Work out the finished part from the listing and answer in its coordinate system (mm). A direction names the side the tool comes from. Give positions to 0.01 mm unless a question says otherwise; leave off trailing zeros. Order: outer loops, then holes, each group sorted by start corner. A loop starts at its lowest first (then second) coordinate and runs counter-clockwise, first axis right, second up. Notation, with made-up numbers: (22, 6.25) - (56, 6.25) arc R15 ccw to (56, 31.25) - close; hole circle Ø1 at (42, -28.75). An arc over 180 degrees is marked (long way). Put each result on its own line as item: value.
Autodesk Inventor part; units mm, degrees
ref_plane "YZ Plane" through (0, 0, 0) normal (1, 0, 0) x (0, 1, 0)
ref_plane "XZ Plane" through (0, 0, 0) normal (0, 1, 0) x (-1, 0, 0)
ref_plane "XY Plane" through (0, 0, 0) normal (0, 0, 1) x (1, 0, 0)
sketch "Эскиз1" plane through (0, 0, 0) normal (0, 0, 1) x (1, 0, 0)
  line L0 (-75.6484, -106.9824) -> (60.0028, -106.9824)
  line L1 (60.0028, 113.8664) -> (-75.6484, 113.8664)
  line L2 (-75.6484, -71.558) -> (-75.6484, 58.442)
  line L3 (60.0028, -71.558) -> (60.0028, 78.442)
  line L4 (63.0028, -109.9824) -> (-78.6484, -109.9824)
  line L5 (-78.6484, -109.9824) -> (-78.6484, 116.8664)
  line L6 (-78.6484, 116.8664) -> (63.0028, 116.8664)
  line L7 (63.0028, 116.8664) -> (63.0028, -109.9824)
  line L8 (60.0028, -106.9824) -> (-75.6484, -106.9824)
  line L9 (-75.6484, -106.9824) -> (-75.6484, 113.8664)
  line L10 (-75.6484, 113.8664) -> (60.0028, 113.8664)
  line L11 (60.0028, 113.8664) -> (60.0028, -106.9824)
  point P0 (0, 0)
  dimension "d0" = 3
  dimension "d1" = 3
  dimension "d2" = 3
  dimension "d3" = 3
extrude "Выдавливание1" add sketch "Эскиз1" along normal blind 60
sketch "Эскиз2" plane through (63.0028, -109.9824, 0) normal (1, 0, 0) x (0, 0, -1)
  point P0 (0, 109.9824)
sketch "Эскиз3" plane through (0, 0, 0) normal (0, 0, -1) x (-1, 0, 0)
  point P0 (0, 0)
sketch "Эскиз4" plane through (63.0028, -109.9824, 0) normal (1, 0, 0) x (0, 0, -1)
  line L0 (-8, 38.4244) -> (-8, 3)
  line L1 (-8, 3) -> (-8, 38.4244)
  line L2 (0.0001, 223.8488) -> (0, 188.4244)
  line L3 (-8, 188.4244) -> (-7.9999, 223.8488)
  line L4 (0, 223.8488) -> (0, 3)
  line L5 (-8, 38.4244) -> (0, 38.4244)
  line L6 (0, 38.4244) -> (0, 3)
  line L7 (0, 3) -> (-8, 3)
  line L8 (-8, 3) -> (-8, 38.4244)
  line L9 (-7.9999, 223.8488) -> (0, 223.8488)
  line L10 (0, 223.8488) -> (0, 188.4244)
  line L11 (0, 188.4244) -> (-7.9999, 188.4244)
  line L12 (-7.9999, 188.4244) -> (-7.9999, 223.8488)
  point P0 (0, 109.9824)
extrude "Выдавливание2" cut sketch "Эскиз4" against normal blind 239.25
sketch "Эскиз5" plane through (0, 0, 60) normal (0, 0, 1) x (1, 0, 0)
  line L0 (73.8028, -108.2777) -> (32.8028, -108.2777)
  line L1 (63.0028, 116.8664) -> (-78.6484, 116.8664)
  line L2 (-78.6484, 116.8664) -> (-78.6484, -109.9824)
  line L3 (-78.6484, -109.9824) -> (63.0028, -109.9824)
  line L4 (63.0028, -109.9824) -> (63.0028, 116.8664)
  line L5 (60.0028, 113.8664) -> (60.0028, -106.9824)
  line L6 (60.0028, -106.9824) -> (-75.6484, -106.9824)
  line L7 (-75.6484, -106.9824) -> (-75.6484, 113.8664)
  line L8 (-75.6484, 113.8664) -> (60.0028, 113.8664)
  line L9 (60.0028, -106.9824) -> (-75.6484, -106.9824)
  line L10 (-75.6484, 113.8664) -> (60.0028, 113.8664)
  line L11 (56.3016, -106.9824) -> (26.1407, -106.9824)
  line L12 (26.1407, -106.9824) -> (26.1407, 113.8664)
  line L13 (26.1407, 113.8664) -> (56.3016, 113.8664)
  line L14 (56.3016, 113.8664) -> (56.3016, -106.9824)
  line L15 (5.2877, -106.9824) -> (-25.8022, -106.9824)
  line L16 (-25.8022, -106.9824) -> (-25.8022, 113.8664)
  line L17 (-25.8022, 113.8664) -> (5.2877, 113.8664)
  line L18 (5.2877, 113.8664) -> (5.2877, -106.9824)
  line L19 (-48.9301, -106.9824) -> (-75.6484, -106.9824)
  line L20 (-75.6484, -106.9824) -> (-75.6484, 111.5008)
  line L21 (-75.6484, 111.5008) -> (-48.9301, 111.5008)
  line L22 (-48.9301, 111.5008) -> (-48.9301, -106.9824)
  line L23 (-75.6484, -106.9824) -> (-75.6484, 113.8664)
  line L24 (-75.6484, -32.9455) -> (-73.4662, -32.9455)
  line L25 (-73.4662, -32.9455) -> (-73.4662, -24.8216)
  line L26 (-73.4662, -24.8216) -> (-75.6484, -24.8216)
  line L27 (-75.6484, -24.8216) -> (-75.6484, -32.9455)
  line L28 (-75.6484, 29.4025) -> (-73.4662, 29.4025)
  line L29 (-73.4662, 29.4025) -> (-73.4662, 36.4767)
  line L30 (-73.4662, 36.4767) -> (-75.6484, 36.4767)
  line L31 (-75.6484, 36.4767) -> (-75.6484, 29.4025)
  point P0 (0, 0)
extrude "Выдавливание3" add sketch "Эскиз5" along normal blind 5 contours L4 L3 L2 L1 | L14 L6 L12 L8 | L18 L6 L16 L8 | L6 L7 L24 L25 L26 L28 L29 L30 L21 L22
sketch "Эскиз6" plane through (0, 0, 65) normal (0, 0, 1) x (1, 0, 0)
  line L0 (-48.9301, 111.5008) -> (-75.6484, 111.5008)
  line L1 (-75.6484, 111.5008) -> (-75.6484, 113.8664)
  line L2 (-48.9301, 111.5008) -> (-75.6484, 111.5008)
  line L3 (-75.6484, 111.5008) -> (-75.6484, 113.8664)
  line L4 (-75.6484, 113.8664) -> (-48.9301, 113.8664)
  line L5 (-48.9301, 113.8664) -> (-48.9301, 111.5008)
  point P0 (0, 0)
extrude "Выдавливание4" add sketch "Эскиз6" against normal blind 5
sketch "Эскиз7" plane through (-78.6484, -71.558, 0) normal (-1, 0, 0) x (0, 0, 1)
  point P0 (0, 71.558)
sketch "Эскиз8" plane through (-78.6484, 116.8664, 0) normal (0, 1, 0) x (1, 0, 0)
  line L0 (85.4799, -9.5) -> (62.4799, -9.5)
  line L1 (74.1362, -4.2225) -> (79.8964, -4.2225)
  line L2 (141.6512, 0) -> (0, 0)
  line L3 (85.4799, -9.5) -> (64.1362, -9.5)
  line L4 (64.1362, -9.5) -> (64.1362, 0)
  line L5 (64.1362, 0) -> (85.4799, 0)
  line L6 (85.4799, 0) -> (85.4799, -9.5)
  line L7 (64.1362, -9.5) -> (89.8964, -9.5)
  line L8 (89.8964, -9.5) -> (89.8964, 0)
  line L9 (89.8964, 0) -> (64.1362, 0)
  line L10 (64.1362, 0) -> (64.1362, -9.5)
  point P0 (78.6484, 0)
  dimension "d12" = 10
  dimension "d13" = 5.584
  dimension "d14" = 10
extrude "Выдавливание5" cut sketch "Эскиз8" against normal blind 5
sketch "Эскиз9" plane through (63.0028, -71.558, 0) normal (1, 0, 0) x (0, 0, -1)
  line L0 (-65, -38.4244) -> (-65, 188.4244)
  arc A0 (-65, 188.4244) -> (-65, -38.4244) centre (307.5062, 75) ccw
  line L1 (0, -38.4244) -> (-65, -38.4244)
  line L2 (-65, -38.4244) -> (-65, -28.4244)
  line L3 (-65, -28.4244) -> (-65, 178.4244)
  arc A1 (-65, 178.4244) -> (-65, -28.4244) centre (307.5062, 75) ccw
  point P0 (0, 71.558)
  dimension "d17" = 10
  dimension "d18" = 10
extrude "Выдавливание6" add sketch "Эскиз9" against normal blind 141.651 contours A0 L0 A1
sketch "Эскиз10" plane through (63.0028, -71.558, 0) normal (1, 0, 0) x (0, 0, -1)
  arc A0 (-65, 178.4244) -> (-65, -28.4244) centre (307.5062, 75) ccw
  line L0 (-65, -28.4244) -> (-65, 178.4244)
  point P0 (0, 71.558)
extrude "Выдавливание7" add sketch "Эскиз10" against normal blind 3
sketch "Эскиз11" plane through (-78.6484, -71.558, 0) normal (-1, 0, 0) x (0, 0, 1)
  arc A0 (65, -28.4244) -> (65, 178.4244) centre (-307.5062, 75) ccw
  line L0 (65, 188.4244) -> (65, -38.4244)
  point P0 (0, 71.558)
extrude "Выдавливание8" add sketch "Эскиз11" against normal blind 3
sketch "Эскиз12" plane through (-78.6484, -109.9824, 0) normal (0, -1, 0) x (1, 0, 0)
  spline S0 degree 3 poles (75.9334, 40.3738) (75.8831, 40.8501) (75.7622, 41.3112) (75.3324, 42.3118) (75.0359, 42.7084) (74.4654, 43.3771) (73.9913, 43.782) (72.8589, 44.371) (72.2642, 44.5465) (71.3446, 44.633) (71.0335, 44.6318) (70.0476, 44.5299) (69.4546, 44.3267) (68.4476, 43.7801) (67.9673, 43.407) (67.0987, 42.3576) (66.8298, 41.785) (66.5793, 40.9818) (66.515, 40.667) (66.4421, 39.9332) (66.4622, 39.6005) (66.486, 39.3756) knots -0.649055 -0.649055 -0.649055 -0.649055 -0.611574 -0.611574 -0.563504 -0.563504 -0.482019 -0.482019 -0.407033 -0.407033 -0.368981 -0.368981 -0.286973 -0.286973 -0.207347 -0.207347 -0.121004 -0.121004 -0.067856 -0.067856 0 0 0 0
  spline S1 degree 3 poles (66.486, 39.3756) (66.5097, 39.1507) (66.5596, 38.8211) (66.7843, 38.1188) (66.913, 37.8244) (67.3257, 37.0912) (67.7084, 36.5875) (68.7772, 35.7428) (69.3247, 35.4783) (70.4238, 35.1543) (71.0461, 35.0795) (72.0316, 35.1858) (72.3361, 35.2497) (73.2173, 35.5265) (73.7622, 35.8224) (74.7465, 36.635) (75.1255, 37.13) (75.5436, 37.9033) (75.7507, 38.353) (75.9619, 39.4214) (75.9837, 39.8976) (75.9334, 40.3738) knots -2.488 -2.488 -2.488 -2.488 -2.22789 -2.22789 -2.024159 -2.024159 -1.693184 -1.693184 -1.387958 -1.387958 -1.073596 -1.073596 -0.927734 -0.927734 -0.640291 -0.640291 -0.327938 -0.327938 -0.143673 -0.143673 0 0 0 0
  point P0 (78.6484, 0)
extrude "Выдавливание9" cut sketch "Эскиз12" against normal blind 3
sketch "Эскиз13" plane through (-78.6484, 116.8664, 65) normal (0, 1, 0) x (1, 0, 0)
  line L0 (49.8619, 5.8292) -> (89.8619, 5.8292)
  line L1 (89.8619, 37.7292) -> (49.8619, 37.7292)
  line L2 (101.9119, 18.2982) -> (101.9119, 14.2982)
  line L3 (101.9119, 29.2602) -> (101.9119, 25.2602)
  line L4 (77.7841, 5.8292) -> (67.7841, 5.8292)
  line L5 (67.7841, 5.8292) -> (67.7841, 2.8292)
  line L6 (67.7841, 2.8292) -> (77.7841, 2.8292)
  line L7 (77.7841, 2.8292) -> (77.7841, 5.8292)
  line L8 (77.7841, 37.7292) -> (67.7841, 37.7292)
  line L9 (67.7841, 37.7292) -> (67.7841, 40.7292)
  line L10 (67.7841, 40.7292) -> (77.7841, 40.7292)
  line L11 (77.7841, 40.7292) -> (77.7841, 37.7292)
  line L12 (111.7909, 14.2982) -> (114.7909, 14.2982)
  line L13 (114.7909, 14.2982) -> (114.7909, 29.2602)
  line L14 (114.7909, 29.2602) -> (111.7909, 29.2602)
  line L15 (111.7909, 29.2602) -> (111.7909, 14.2982)
  point P0 (78.6484, 65)
  point P1 (67.7841, 5.8292)
  dimension "d27" = 10
  dimension "d28" = 3
  dimension "d29" = 3
  dimension "d30" = 3
extrude "Выдавливание10" cut sketch "Эскиз13" against normal blind 3
sketch "Эскиз14" plane through (-78.6484, 116.8664, 65) normal (0, 1, 0) x (1, 0, 0)
  circle A0 centre (26.4286, 24.6652) radius 8
  circle A1 centre (47.4286, 24.6652) radius 8
  point P0 (78.6484, 65)
  dimension "d33" = 16
  dimension "d45" = 16
  dimension "d46" = 21
extrude "Выдавливание11" cut sketch "Эскиз14" against normal blind 3
chamfer "Фаска1" distance 2 angle 45 1 edges at (-60.2198, 116.8664, 40.3348)
sketch "Эскиз15" plane through (-78.6484, -71.558, 0) normal (-1, 0, 0) x (0, 0, 1)
  line L0 (-6, 73) -> (-6, 77)
  line L1 (-6, 73) -> (-6, 77)
  circle A0 centre (10, 75) radius 1.5
  line L2 (0, 150) -> (0, 0)
  point P0 (0, 71.558)
  dimension "d39" = 3
  dimension "d40" = 10
extrude "Выдавливание12" cut sketch "Эскиз15" against normal blind 560
sketch "Эскиз16" plane through (0, 0, 0) normal (0, 0, -1) x (-1, 0, 0)
  line L0 (75.6484, -71.558) -> (78.6484, -71.558)
  line L1 (78.6484, 78.442) -> (78.6484, -71.558)
  line L2 (78.6484, 78.442) -> (75.6484, 78.442)
  line L3 (75.6484, -71.558) -> (75.6484, 78.442)
  line L4 (-63.0028, -71.558) -> (-60.0028, -71.558)
  line L5 (-60.0028, 78.442) -> (-60.0028, -71.558)
  line L6 (-60.0028, 78.442) -> (-63.0028, 78.442)
  line L7 (-63.0028, -71.558) -> (-63.0028, 78.442)
  line L8 (78.6484, -106.9824) -> (-63.0028, -106.9824)
  line L9 (-63.0028, -109.9824) -> (-63.0028, -106.9824)
  line L10 (78.6484, -109.9824) -> (-63.0028, -109.9824)
  line L11 (78.6484, -106.9824) -> (78.6484, -109.9824)
  line L12 (-11.248, 113.8664) -> (-11.248, 116.8664)
  line L13 (-63.0028, 116.8664) -> (-11.248, 116.8664)
  line L14 (-63.0028, 113.8664) -> (-63.0028, 116.8664)
  line L15 (-63.0028, 113.8664) -> (-11.248, 113.8664)
  line L16 (14.5122, 116.8664) -> (14.5122, 113.8664)
  line L17 (14.5122, 113.8664) -> (78.6484, 113.8664)
  line L18 (78.6484, 116.8664) -> (78.6484, 113.8664)
  line L19 (14.5122, 116.8664) -> (78.6484, 116.8664)
  point P0 (0, 0)
extrude "Выдавливание13" add sketch "Эскиз16" along normal blind 6
chamfer "Фаска2" distance 2 angle 45 1 edges at (-39.2198, 116.8664, 40.3348)
equation "\"d2\" = d1"
equation "\"d3\" = d0"
properties part number "3Dkrish"
(1) Given pin 1 (0.9 mm diameter, centred on x = 61, y = -90, fed in from -Z); pin 2 (1.5 mm diameter, centred on x = -3.5, y = 115.5, fed in from -Z); pin 3 (5 mm diameter, centred on x = 17, y = 49.5, fed in from -Z), each flat-ended and moving along its own axis, determine where each tip first touches the part or whether it passes through.
Geometry check:
pin 1: stops at z = 8
pin 2: stops at z = 9.5
pin 3: stops at z = 76.03
(2) Section D-D, the plane x = 23 is taken. Write down the section's boundary in (y, z), then the cut area to 3 significant figures.
Geometry check:
outline: (-109.98, -6) - (-106.98, -6) - (-106.98, 65) - (-99.98, 65) arc R386.6 cw to (106.87, 65) - (113.87, 65) - (113.87, -6) - (116.87, -6) - (116.87, 65) arc R389.39 ccw to (-109.98, 65) - close
area: 1,040 mm²
(3) A tool of negligible diameter and unlimited length cuts with its end or side. For faces 4 (the face through (-78.648, 12, 80)), 5 (the face through (-48.93, 5, 63)), 6 (the face through (-37.57, 114.37, 45.2)), from which of +Z, -Z, +X, -X, +Y, -Y can it reach the whole face along a straight path? Write none if from no direction.
Geometry check:
face 4: +Z, -Z, -X, +Y, -Y
face 5: -Z
face 6: +Y
(4) Section A-A, the plane z = 5.5 is taken. Write down the section's boundary in (x, y), then the cut area to 3 significant figures.
Geometry check:
outline: (-78.65, -109.98) - (63, -109.98) - (63, -106.98) - (-78.65, -106.98) - close; (-78.65, -71.56) - (-75.65, -71.56) - (-75.65, 78.44) - (-78.65, 78.44) - close; (-78.65, 113.87) - (-14.51, 113.87) - (-14.51, 116.87) - (-78.65, 116.87) - close; (11.25, 113.87) - (63, 113.87) - (63, 116.87) - (11.25, 116.87) - close; (60, -71.56) - (63, -71.56) - (63, 78.44) - (60, 78.44) - close
area: 1,670 mm²
(5) Section C-C, the plane x = -70 is taken. Write down the section's boundary in (y, z).
Geometry check:
outline: (-109.98, -6) - (-106.98, -6) - (-106.98, 60) - (113.87, 60) - (113.87, -6) - (116.87, -6) - (116.87, 65) arc R389.39 ccw to (-109.98, 65) - close; hole (-99.98, 65) - (106.87, 65) arc R386.6 ccw to start
(6) Straight lines are drawn through the part: line 1 (X direction, y = -96, z = 21.5); line 2 (Y direction, x = -63, z = 55); line 3 (Z direction, x = -64.5, y = 6). For each, find the intervals that lie inside material, in ascending order.
Geometry check:
line 1: x = -78.65 to -75.65, 60 to 63
line 2: y = -109.98 to -106.98, 113.87 to 116.87
line 3: z = 60 to 65, 79.08 to 81.88
(7) Section B-B, the plane y = -74 is taken. Count the separate pieces of the cut face and the enclosed holes in it, then the cut area to 3 significant figures.
Geometry check:
separate pieces: 3
enclosed holes: 0
area: 1,220 mm²
(8) Determine the mould class of faces 1 (the face through (-6.87, 4.91, 79.09)), 2 (the face through (-48.47, 114.99, 47.54)), 3 (the face through (-53.954, 114.373, 48.145)) for opening direction Y: pulls with the +Y half, pulls with the -Y half, needs draft (parallel to the pull), parting line crosses it, or undercut.
Geometry check:
face 1: undercut
face 2: pulls with the +Y half
face 3: needs draft
